Autodesk Inventor part; units mm, degrees
ref_plane "YZ Plane" through (0, 0, 0) normal (1, 0, 0) x (0, 1, 0)
ref_plane "XZ Plane" through (0, 0, 0) normal (0, 1, 0) x (-1, 0, 0)
ref_plane "XY Plane" through (0, 0, 0) normal (0, 0, 1) x (1, 0, 0)
sketch "Sketch1" plane through (0, 0, 0) normal (0, 0, 1) x (1, 0, 0)
  line L0 (-35.1442, 12.6555) -> (24.8558, 12.6555)
  line L1 (24.8558, 12.6555) -> (24.8558, -7.3445)
  line L2 (24.8558, -7.3445) -> (-35.1442, -7.3445)
  line L3 (-35.1442, -7.3445) -> (-35.1442, 12.6555)
  point P0 (0, 0)
  dimension "d0" = 60
  dimension "d1" = 20
extrude "Extrusion1" add sketch "Sketch1" along normal blind 20
sketch "Sketch2" plane through (-35.1442, 12.6555, 0) normal (0, 1, 0) x (1, 0, 0)
  line L0 (0, 0) -> (0, -20)
  line L1 (60, 0) -> (60, -20)
  line L2 (0, 0) -> (60, 0)
  circle A0 centre (10, -10) radius 3.5
  circle A1 centre (50, -10) radius 3.5
  point P0 (35.1442, 0)
  dimension "d4" = 40
  dimension "d5" = 10
  dimension "d6" = 10
  dimension "d7" = 10
  dimension "d8" = 7
  dimension "d9" = 7
extrude "Extrusion2" cut sketch "Sketch2" against normal blind 20
sketch "Sketch3" plane through (0, 0, 20) normal (0, 0, 1) x (1, 0, 0)
  line L0 (-35.1442, 12.6555) -> (24.8558, 12.6555)
  line L1 (-35.1442, 12.6555) -> (-35.1442, -7.3445)
  line L2 (24.8558, -7.3445) -> (24.8558, 12.6555)
  point P0 (0, 0)
  point P1 (-17.6442, 2.6555)
  point P2 (7.3558, 2.6555)
  dimension "d12" = 10
  dimension "d13" = 10
  dimension "d14" = 25
  dimension "d15" = 17.5
  dimension "d16" = 17.5
hole "Hole1" at (-17.6442, 2.6555, 20) at (7.3558, 2.6555, 20) direction (0, 0, -1) diameter 3 depth 8 tip angle 118
sketch "Sketch4" plane through (-35.1442, 12.6555, 0) normal (0, 1, 0) x (1, 0, 0)
  line L0 (60, 0) -> (0, 0)
  line L1 (16, 0) -> (44, 0)
  line L2 (44, 0) -> (44, -6)
  line L3 (44, -6) -> (16, -6)
  line L4 (16, -6) -> (16, 0)
  line L5 (0, 0) -> (0, -20)
  line L6 (60, 0) -> (60, -20)
  point P0 (35.1442, 0)
  dimension "d24" = 16
  dimension "d25" = 16
  dimension "d26" = 6
extrude "Extrusion3" cut sketch "Sketch4" against normal blind 20
chamfer "Chamfer1" distance 6 angle 45 2 edges at (8.8558, 2.6555, 0) (-19.1442, 2.6555, 0)
sketch "Sketch5" plane through (-35.1442, 12.6555, 20) normal (0, 1, 0) x (1, 0, 0)
  point P0 (35.1442, 20)
sketch "Sketch6" plane through (8.8558, 12.6555, 6) normal (0, 0, -1) x (-1, 0, 0)
  point P0 (8.8558, -12.6555)
sketch "Sketch7" plane through (-35.1442, 12.6555, 20) normal (0, 1, 0) x (1, 0, 0)
  line L0 (20, 20) -> (40, 20)
  line L1 (40, 20) -> (40, 17.5)
  line L2 (40, 17.5) -> (20, 17.5)
  line L3 (20, 17.5) -> (20, 20)
  line L4 (0, 20) -> (0, 0)
  line L5 (60, 20) -> (60, 0)
  line L6 (50, 20) -> (60, 20)
  line L7 (44, 14) -> (16, 14)
  line L8 (27, 14) -> (33, 14)
  line L9 (33, 14) -> (33, 17.5)
  line L10 (33, 17.5) -> (27, 17.5)
  line L11 (27, 17.5) -> (27, 14)
  point P0 (35.1442, 20)
  dimension "d32" = 20
  dimension "d33" = 20
  dimension "d34" = 2.5
  dimension "d35" = 7
  dimension "d36" = 7
extrude "Extrusion4" add sketch "Sketch7" against normal blind 20
chamfer "Chamfer2" distance 3 angle 45 2 edges at (-5.1442, 12.6555, 0) (-5.1442, -7.3445, 0)
chamfer "Chamfer3" distance 5 angle 45 2 edges at (24.8558, 2.6555, 0) (-35.1442, 2.6555, 0)
sketch "Sketch8" plane through (4.8558, -4.3445, 0) normal (0, 0, -1) x (-1, 0, 0)
  line L0 (10, 3.5052) -> (12.1213, 5.6266)
  line L1 (10, 3.5052) -> (13, 3.5052) construction
  line L2 (12.1213, 5.6266) -> (7.8787, 5.6266)
  line L3 (7.8787, 5.6266) -> (10, 3.5052)
  point P0 (4.8558, 4.3445)
  dimension "d45" = 3
  dimension "d46" = 45
extrude "Extrusion5" cut sketch "Sketch8" against normal blind 1
properties part number "Moving block"
Check sheet for the modelled part. Datum: model origin and axes. Units: mm. A direction names the side the tool comes from. Round coordinates to 2 decimals unless told otherwise and drop trailing zeros. Write each loop counter-clockwise with the first axis right and the second up, starting at its lowest first coordinate (ties: lowest second). Pieces come first, ordered by that corner, then holes. Notation, with made-up numbers: M -11,76 L 42,76 A29 cw 42,112 Z; hole C -6.5,-0.75 d11. An arc over 180 degrees is marked long. Write item = value, one per line. Start each with the question number.
1. Scan lines: line 1 (X direction, y = -3, z = 9.75); line 2 (X direction, y = -3.5, z = 10); line 3 (Z direction, x = 3.5, y = 8.25). Record each from-to range of solid material in increasing order. Write a range as [from, to].
2. Gauge pin test, flat ends, axial feed: pin 1 (5.5 mm diameter, centred on x = -25.14, z = 10, fed in from -Y); pin 2 (1.3 mm diameter, centred on y = 4.5, z = 0.5, fed in from -X); pin 3 (2.5 mm diameter, centred on x = -17.64, y = 2.66, fed in from +Z); pin 4 (0.8 mm diameter, centred on y = -2, z = 1, fed in from +X). Record the tip position at first contact, or that the pin passes through.
3. Section check C-C, the plane x = 0.5. Record the cut outline in (y, z), then the cut area to 3 significant figures.
4. Tool access check on faces 4 (the flat face through (-28, 3, 0)), 5 (the flat face through (-5.004, 11.134, 1.479)), 6 (the flat face through (-12, 3, 2.5)), 7 (the flat face through (11.898, 2.795, 2.958)), 8 (the cylindrical face through (5.87, 2.85, 15.94)). Record the directions out of +Z, -Z, +X, -X, +Y, -Y that give a thin tool (end or side, any length) a straight path to the whole face; none if there is none.
5. Release check for a two-part mould opening along Z. For faces 1 (the flat face through (-2.144, 3, 4)), 2 (the flat face through (17, 3, 0)), 3 (the flat face through (-5, -7.344, 12)) record: pulls with the +Z half, pulls with the -Z half, needs draft (parallel to the pull), parting line crosses it, or undercut.
6. Section check B-B, the plane y = 6.25. State how many separate pieces and enclosed holes the cut face has, then the cut area to 3 significant figures.
7. Section check D-D, the plane x = -6. Record the cut outline in (y, z), then the cut area to 3 significant figures.
8. Section check A-A, the plane z = 10. Record the cut outline in (x, y), then the cut area to 3 significant figures.
Results found:
q1.line_1 = [-35.14, -28.64], [-21.65, 11.36], [18.35, 24.86]
q1.line_2 = [-35.14, -28.64], [-21.64, 11.36], [18.36, 24.86]
q1.line_3 = [0, 2.5], [6, 20]
q2.pin_1 = through
q2.pin_2 = -31.29
q2.pin_3 = 11.85
q2.pin_4 = 21.26
q3.outline = M -7.34,6 L 12.66,6 L 12.66,20 L -7.34,20 Z; M -6.84,2.5 L -4.34,0 L 9.66,0 L 12.16,2.5 Z
q3.area = 321 mm^2
q4.face_4 = -Z, +X, -X, +Y, -Y
q4.face_5 = -Z, +Y
q4.face_6 = +Y, -Y
q4.face_7 = -Z, +Y, -Y
q4.face_8 = +Z
q5.face_1 = undercut
q5.face_2 = pulls with the -Z half
q5.face_3 = needs draft
q6.separate_pieces = 1
q6.enclosed_holes = 2
q6.area = 965 mm^2
q7.outline = M -7.34,3 L -4.34,0 L 0.02,0 L 0.02,1 L 1.28,1 L 1.28,0 L 9.66,0 L 12.66,3 L 12.66,20 L -7.34,20 Z
q7.area = 390 mm^2
q8.outline = M -35.14,-7.34 L -28.64,-7.34 L -28.64,12.66 L -35.14,12.66 Z; M -21.64,-7.34 L 11.36,-7.34 L 11.36,12.66 L -21.64,12.66 Z; M 18.36,-7.34 L 24.86,-7.34 L 24.86,12.66 L 18.36,12.66 Z
q8.area = 920 mm^2
